from build123d import *

# Parameters (mm, degrees)
F2_R   = 410.9
F2_R_2 = 400


with BuildPart() as f3:
    # F3: sweep along a path in F0
    with BuildLine(Plane.XZ) as f3_path:
        Line((-46, 800), (331.3708498985, 800))
        Line((331.3708498985, 800), (800, 331.3708498985))
        Line((800, 331.3708498985), (800, -46))
    # F2 (on line) → F3 (sweep)
    with BuildSketch(Plane.YZ.offset(-46)):
        with Locations((0, 800)):
            Circle(F2_R)
        with Locations((0, 800)):
            Circle(F2_R_2, mode=Mode.SUBTRACT)
    sweep(path=f3_path.line, transition=Transition.RIGHT)


solid = f3.part
Can you work these out from the model? Positions are in its coordinate system, mm. A direction names the side the tool comes from. Coordinates: 2 decimals unless noted, no trailing zeros. Order: outer loops, then holes, each group sorted by start corner. A loop starts at its lowest first (then second) coordinate and runs counter-clockwise, first axis right, second up. Notation, with made-up numbers: (7, -18) - (64, -18) arc R22 cw to (64, -9) - close; hole circle Ø4 at (-11.5, 13.5). An arc over 180 degrees is marked (long way). Answer as a JSON object with one key per item and string values. Group by question number.
Q1. Imagine slicing it at C-C (z = 132). Please give me the cut outline in (x, y).
Q2. Will these pins go through, and if not, where does the flat tip stop? P1, Ø6, axis at x = 354.5, z = 973.5, coming from the +Y side; P2, Ø12, axis at x = 898.5, y = 196.5, coming from the -Z side; P3, Ø5, axis at y = -150.5, z = 733.5, coming from the -X side.
Q3. Imagine slicing it at B-B (y = -213). Please give me the cut outline in (x, z), and give its area (3 significant figures).
Q4. On a 3-axis mill with a long thin cutter (end or side, diameter ignored), from which of +Z, -Z, +X, -X, +Y, -Y can I reach the whole of each face in a straight line? I mean faces 1 (the face through (170.777, -53.491, 1207.403)), 2 (the face through (851.042, -52.072, 841.201)), 3 (the face through (1207.403, -53.491, 163.111)). Say none if no direction works.
Q5. We'd pull the mould along X, two halves only. Please class faces 4 (the face through (1196.596, -52.072, 161.387)), 5 (the face through (-46, 394, 889)), 6 (the face through (858.728, -53.491, 848.798)), 7 (the face through (711, -394, -46)): +X half, -X half, draft (parallel to the pull), parting line (faces both ways), or undercut.
Q6. I need wall thicknesses on line 1 (Z direction, x = 88, y = 0); line 2 (X direction, y = 13.5, z = 142); line 3 (Y direction, x = 935.5, z = 163.5). Which ranges of each line are inside material? Lowest first, please. Write a range as from..to.
Q7. Imagine slicing it at A-A (y = 0). Please give me the cut outline in (x, z).
Determined:
{
 "1": {"outline": "circle Ø821.8 at (800, 0); hole circle Ø800 at (800, 0)"},
 "2": {"P1": "stops at y = 373.86", "P2": "stops at z = 717.88", "P3": "stops at x = 919.1"},
 "3": {"outline": "(-46, 448.62) - (185.82, 448.62) - (448.62, 185.82) - (448.62, -46) - (461.43, -46) - (461.43, 191.13) - (191.13, 461.43) - (-46, 461.43) - close; (-46, 1138.57) - (471.61, 1138.57) - (1138.57, 471.61) - (1138.57, -46) - (1151.38, -46) - (1151.38, 476.92) - (476.92, 1151.38) - (-46, 1151.38) - close", "area": "36,300 mm2"},
 "4": {"face 1": "-X", "face 2": "none", "face 3": "-Z"},
 "5": {"face 4": "undercut", "face 5": "-X half", "face 6": "parting line", "face 7": "draft"},
 "6": {"line 1": "z = 389.1..400, 1200..1210.9", "line 2": "x = 389.32..400.23, 1199.77..1210.68", "line 3": "y = -387.92..-376.35, 376.35..387.92"},
 "7": {"outline": "(-46, 389.1) - (161.17, 389.1) - (389.1, 161.17) - (389.1, -46) - (400, -46) - (400, 165.69) - (165.69, 400) - (-46, 400) - close; (-46, 1200) - (497.06, 1200) - (1200, 497.06) - (1200, -46) - (1210.9, -46) - (1210.9, 501.57) - (501.57, 1210.9) - (-46, 1210.9) - close"}
}
